Source: CAD feature listing. Evaluate the final solid. Frame: model axes, mm. Face numbers are marked on the shaded views. A direction names the side the tool comes from. Coordinates: 2 decimals unless noted, no trailing zeros. Order: outer loops, then holes, each group sorted by start corner. A loop starts at its lowest first (then second) coordinate and runs counter-clockwise, first axis right, second up.
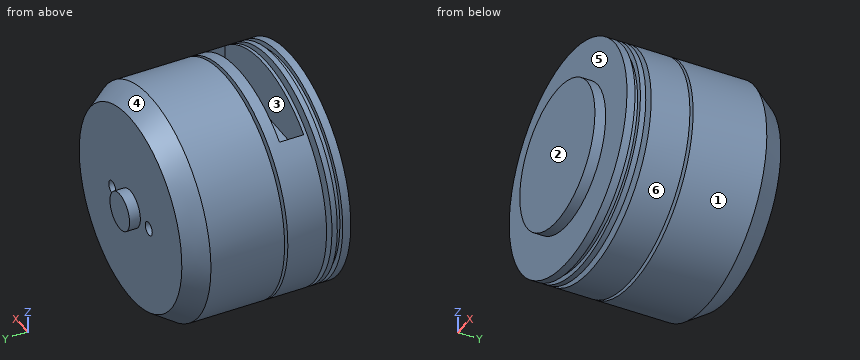
```python
from build123d import *

# Parameters (mm, degrees)
SKETCH_2_W             = 28
SKETCH_2_H             = 4.5
CUT_EXTRUDE_1_DEPTH    = 10
HOLE_WIZARD_M3_1_D     = 2.5
HOLE_WIZARD_M3_1_DEPTH = 4
HOLE_WIZARD_M3_1_TIP   = 0.751075774
SKETCH_18_R            = 3.5
CUT_EXTRUDE_3_DEPTH    = 3
CUT_EXTRUDE_START      = -6.7
SKETCH_19_R            = 4.1
CUT_EXTRUDE_4_DEPTH    = 6.7


with BuildPart() as part:
    # 草图1 → 旋转1 (revolve)
    with BuildSketch(Plane.XY, mode=Mode.PRIVATE) as revolve_1_sk:
        Polygon((0, 0), (4.1, 0), (4.1, 6.7), (13.4, 6.7), (13.4, 8.7), (21, 8.7), (21, 10.2), (20, 10.2), (20, 11.2), (21, 11.2), (21, 12.2), (10, 12.2), (10, 13.2), (21, 13.2), (21, 20.4), (5, 20.4), (5, 21), (21, 21), (21, 34.7), (18.3, 38.7), (3.5, 38.7), (3.5, 43.7), (0, 43.7), align=None)
    revolve(revolve_1_sk.sketch.rotate(Axis((0, 43.7, 0), (0, -1, 0)), 90), axis=Axis((0, 43.7, 0), (0, -1, 0)))

    # 草图2 → 切除-拉伸1 (cut)
    with BuildSketch(Plane.XY.offset(21)):
        with Locations((0, 16.05)):
            Rectangle(SKETCH_2_W, SKETCH_2_H)
    extrude(amount=-CUT_EXTRUDE_1_DEPTH, mode=Mode.SUBTRACT)

    # M3 螺纹孔1
    with Locations(Plane(origin=(0, 38.7, 0), x_dir=(1, 0, 0), z_dir=(0, 1, 0))):
        with Locations((-6.5, 0), (6.5, 0)):
            Hole(HOLE_WIZARD_M3_1_D / 2, depth=HOLE_WIZARD_M3_1_DEPTH)
            with Locations((0, 0, -(HOLE_WIZARD_M3_1_DEPTH + HOLE_WIZARD_M3_1_TIP / 2))):  # 118° drill point
                Cone(0, HOLE_WIZARD_M3_1_D / 2, HOLE_WIZARD_M3_1_TIP, mode=Mode.SUBTRACT)

    # 草图18 → 切除-拉伸3 (cut)
    with BuildSketch(Plane(origin=(0, 43.7, 0), x_dir=(1, 0, 0), z_dir=(0, 1, 0))):
        with Locations(Location((0, 0, 0), (0, 0, 270))):
            Circle(SKETCH_18_R)
    extrude(amount=-CUT_EXTRUDE_3_DEPTH, mode=Mode.SUBTRACT)

    # 草图19 → 切除-拉伸4 (cut)
    with BuildSketch(Plane.XZ.offset(CUT_EXTRUDE_START)):
        Circle(SKETCH_19_R)
    extrude(amount=CUT_EXTRUDE_4_DEPTH, mode=Mode.SUBTRACT)


solid = part.part
```
Q1. Set-up query: the marked faces 5 and 6. Return all of +Z, -Z, +X, -X, +Y, -Y with unobstructed straight access to the full face (end or side cutting, diameter ignored); none if empty.
Solutions:
face 5: -Y
face 6: +Y, -Y
Q2. Pull-direction query (Y, two-part tool) for the marked faces 1, 2, 3 and 4; classes: pulls with the +Y half, pulls with the -Y half, needs draft (parallel to the pull), parting line crosses it, or undercut.
Solutions:
face 1: needs draft
face 2: pulls with the -Y half
face 3: undercut
face 4: pulls with the +Y half
Q3. Pin query (flat end, axial travel): P1, Ø3.5, axis at x = -1, y = 16, coming from the +Z side; P2, Ø2, axis at x = -10, y = 23, coming from the -Z side; P3, Ø5, axis at x = 16, z = -9, coming from the -Y side; P4, Ø12.5, axis at x = -2, z = -5.5, coming from the +Y side. Return the tip coordinate at first contact, or that it passes through.
Solutions:
P1: stops at z = 11
P2: stops at z = -18.97
P3: stops at y = 8.7
P4: stops at y = 40.7
Q4. Material intervals for line 1 along Y through (x, z) = (-15.5, -2); line 2 along Y through (x, z) = (-9.5, 3.5); line 3 along Y through (x, z) = (-7, 16.5), sorted ascending.
Solutions:
line 1: y = 8.7 to 12.2, 13.2 to 20.4, 21 to 38.7
line 2: y = 6.7 to 12.2, 13.2 to 20.4, 21 to 38.7
line 3: y = 8.7 to 12.2, 13.2 to 13.8, 18.3 to 20.4, 21 to 38.7
Q5. Section query A-A on y = 16. Output: boundary loops of the cut face in (x, z), plus the area to 3 significant figures.
Solutions:
outline: (-14, 11) - (-14, 15.65) arc R21 ccw (long way) to (14, 15.65) - (14, 11) - close
area: 1,150 mm2
Q6. Section query B-B on z = 12.5. Give the number of separate pieces and of enclosed holes in the cut face, plus the area to 3 significant figures.
Solutions:
separate pieces: 3
enclosed holes: 1
area: 835 mm2
